Geometry: final body of the model. Coordinates: model frame, mm. Give positions to 0.01 mm unless a question says otherwise; leave off trailing zeros. Write each loop counter-clockwise with the first axis right and the second up, starting at its lowest first coordinate (ties: lowest second). Pieces come first, ordered by that corner, then holes. Notation, with made-up numbers: M -26,49 L 6,49 A17 ccw 6,57 Z; hole C 70.5,11.25 d6. An arc over 180 degrees is marked long. Use a Markdown table: item, result. Add a question column.
(1) Material intervals for L1, parallel to Z at x = 2.25, y = 0.45; L2, parallel to Z at x = 0, y = 0.9; L3, parallel to Y at x = 4.25, z = 7, sorted ascending.
(2) Cut plane C-C (y = 0.8). Output: boundary loops of the cut face in (x, z).
(3) Draft query along Y for faces 1 (the flat face through (0, 0, 0)), 2 (the flat face through (0, 0.5, 7)). Return one class per face: released by +Y, released by -Y, zero draft, split by the parting line, or undercut.
(4) Cut plane D-D (y = -0.65). Output: boundary loops of the cut face in (x, z).
(5) Cut plane A-A (z = 2.5). State how many separate pieces and enclosed holes the cut face has, plus the area to 3 significant figures.
Autodesk Inventor part; units mm, degrees
ref_plane "YZ Plane" through (0, 0, 0) normal (1, 0, 0) x (0, 1, 0)
ref_plane "XZ Plane" through (0, 0, 0) normal (0, 1, 0) x (-1, 0, 0)
ref_plane "XY Plane" through (0, 0, 0) normal (0, 0, 1) x (1, 0, 0)
sketch "Sketch1" plane through (0, 0, 0) normal (0, 0, 1) x (1, 0, 0)
  line L0 (-4.5, -1.5) -> (4.5, -1.5)
  line L1 (4.5, -1.5) -> (4.5, 1.5)
  line L2 (4.5, 1.5) -> (-4.5, 1.5)
  line L3 (-4.5, 1.5) -> (-4.5, -1.5)
  point P0 (0, 0)
  dimension "d0" = 3
  dimension "d1" = 1.5
  dimension "d2" = 9
  dimension "d3" = 4.5
extrude "Extrusion1" add sketch "Sketch1" along normal blind 10.5
fillet "Fillet1" radius 1.5 4 edges at (4.5, 1.5, 5.25) (4.5, -1.5, 5.25) (-4.5, -1.5, 5.25) (-4.5, 1.5, 5.25)
sketch "Sketch2" plane through (0, 0, 10.5) normal (0, 0, 1) x (1, 0, 0)
  arc A0 (-3, 1.5) -> (-3, -1.5) centre (-3, 0) ccw
  line L0 (-3, -1.5) -> (3, -1.5)
  arc A1 (3, -1.5) -> (3, 1.5) centre (3, 0) ccw
  line L1 (3, 1.5) -> (-3, 1.5)
  arc A2 (-3, 1.4) -> (-3, -1.4) centre (-3, 0) ccw
  line L2 (-3, 1.4) -> (3, 1.4)
  arc A3 (3, -1.4) -> (3, 1.4) centre (3, 0) ccw
  line L3 (3, -1.4) -> (-3, -1.4)
  point P0 (0, 0)
  dimension "d7" = 0.1
extrude "Extrusion2" cut sketch "Sketch2" against normal blind 10 contours L2 A3 L3 A2
sketch "Sketch4" plane through (-3, 1.5, 0) normal (0, 1, 0) x (1, 0, 0)
  line L0 (2.5, -8.5) -> (2.025, -6.6503)
  line L1 (1.8313, -6.5) -> (1.6687, -6.5)
  line L2 (1.475, -6.6503) -> (1, -8.5)
  line L3 (6, -10.5) -> (0, -10.5)
  arc A0 (1.6687, -6.5) -> (1.475, -6.6503) centre (1.6687, -6.7) ccw
  arc A1 (2.025, -6.6503) -> (1.8313, -6.5) centre (1.8313, -6.7) ccw
  line L4 (2.3545, -8.5) -> (1.8886, -6.6853)
  arc A2 (1.8886, -6.6853) -> (1.8313, -6.6409) centre (1.8313, -6.7) ccw
  line L5 (1.8313, -6.6409) -> (1.6687, -6.6409)
  arc A3 (1.6687, -6.6409) -> (1.6114, -6.6853) centre (1.6687, -6.7) ccw
  line L6 (1.6114, -6.6853) -> (1.1455, -8.5)
  line L7 (1, -8.5) -> (1.1455, -8.5)
  line L8 (2.3545, -8.5) -> (2.5, -8.5)
  point P0 (3, 0)
  point P1 (1.9865, -6.5)
  point P2 (1.5135, -6.5)
  dimension "d11" = 0.5135
  dimension "d12" = 0.5135
  dimension "d13" = 1.5
  dimension "d14" = 2
  dimension "d15" = 2
  dimension "d16" = 1
  dimension "d17" = 0.4729
  dimension "d18" = 0.2
extrude "Extrusion3" cut sketch "Sketch4" against normal blind 1
mirror "Mirror2" about plane through (0, 0, 0) normal (1, 0, 0) of "Extrusion3"
sketch "Sketch5" plane through (0, 0, 0.5) normal (0, 0, 1) x (1, 0, 0)
  arc A0 (-3, 1.4) -> (-3, -1.4) centre (-3, 0) ccw
  line L0 (3, -1.4) -> (-3, -1.4)
  arc A1 (3, -1.4) -> (3, 1.4) centre (3, 0) ccw
  line L1 (-3, 1.4) -> (3, 1.4)
  arc A2 (-3, 1.35) -> (-3, -1.35) centre (-3, 0) ccw
  line L2 (-3, 1.35) -> (3, 1.35)
  arc A3 (3, -1.35) -> (3, 1.35) centre (3, 0) ccw
  line L3 (3, -1.35) -> (-3, -1.35)
  point P0 (0, 0)
  dimension "d21" = 0.05
extrude "Extrusion4" add sketch "Sketch5" along normal blind 4 contours L2 A3 L3 A2
sketch "Sketch6" plane through (0, 0, 4.5) normal (0, 0, 1) x (1, 0, 0)
  line L0 (-3, 0.5) -> (3, 0.5)
  line L1 (3, 0.5) -> (3, -0.5)
  line L2 (3, -0.5) -> (-3, -0.5)
  line L3 (-3, -0.5) -> (-3, 0.5)
  point P0 (0, 0)
  dimension "d24" = 1
  dimension "d25" = 0.5
  dimension "d26" = 6
  dimension "d27" = 3
extrude "Extrusion5" add sketch "Sketch6" along normal blind 5
fillet "Fillet2" radius 0.3 4 edges at (-3, 0.5, 7) (-3, -0.5, 7) (3, 0.5, 7) (3, -0.5, 7)
properties part number "XGEN_USB-C_socket_pcb"
Answer list:
| question | item | result |
|---|---|---|
| 1 | L1 | 0 to 9.5 |
| 1 | L2 | 0 to 4.5 |
| 1 | L3 | -0.83 to -0.63, 0.63 to 0.83 |
| 2 | outline | M -4.27,0 L 4.27,0 L 4.27,10.5 L 4.15,10.5 L 4.15,0.5 L 4.09,0.5 L 4.09,4.5 L -4.09,4.5 L -4.09,0.5 L -4.15,0.5 L -4.15,10.5 L -4.27,10.5 Z |
| 3 | face 1 | zero draft |
| 3 | face 2 | undercut |
| 4 | outline | M -4.35,0 L 4.35,0 L 4.35,10.5 L 4.24,10.5 L 4.24,0.5 L 4.18,0.5 L 4.18,4.5 L -4.18,4.5 L -4.18,0.5 L -4.24,0.5 L -4.24,10.5 L -4.35,10.5 Z |
| 5 | separate pieces | 2 |
| 5 | enclosed holes | 1 |
| 5 | area | 24.0 mm² |
